Source: CAD feature listing. Evaluate the final solid. Frame: model axes, mm. Give positions to 0.01 mm unless a question says otherwise; leave off trailing zeros. Use CSV: the item, a comma, the result in double quotes.
```python
from build123d import *

# Parameters (mm, degrees)
EXTRUDE_1_DEPTH     = 15
SKETCH_2_R          = 0.75
CUT_EXTRUDE_1_DEPTH = 15
SKETCH_3_R          = 0.75
CUT_EXTRUDE_2_DEPTH = 15
CUT_EXTRUDE_START   = -2.7
SKETCH_2_2_R        = 0.75
CUT_EXTRUDE_3_DEPTH = 1
CUT_EXTRUDE_3_TAPER = -60
CUT_EXTRUDE_START_2 = 2.7
SKETCH_3_2_R        = 0.75
CUT_EXTRUDE_4_DEPTH = 1
CUT_EXTRUDE_4_TAPER = -60
FILLET_1_R          = 0.5


with BuildPart() as part:
    # Sketch 1 → Extrude 1 (new body)
    with BuildSketch(Plane(origin=(0, 0, 0), x_dir=(0, 0, -1), z_dir=(1, 0, 0))):
        with BuildLine():
            Line((0, 0), (-3, 0))
            Line((-3, 0), (-3, -20))
            Line((-3, -20), (-10.878462024, -21.389185421))
            Line((-10.878462024, -21.389185421), (-10.357517491, -24.34360868))
            Line((-10.357517491, -24.34360868), (-2.479055467, -22.954423259))
            ThreePointArc((-2.479055467, -22.954423259), (-0.701866671, -21.928362829), (0, -20))
            Line((0, -20), (0, 0))
        make_face()
    extrude(amount=EXTRUDE_1_DEPTH)

    # Sketch 2 → Cut-Extrude 1 (cut)
    with BuildSketch(Plane.XY.offset(3)):
        with Locations((2, -3)):
            Circle(SKETCH_2_R)
        with Locations((5.666666667, -3)):
            Circle(SKETCH_2_R)
        with Locations((9.333333333, -3)):
            Circle(SKETCH_2_R)
        with Locations((13, -3)):
            Circle(SKETCH_2_R)
        with Locations((3.680498092, -5.4)):
            Circle(SKETCH_2_R)
        with Locations((7.347164758, -5.4)):
            Circle(SKETCH_2_R)
        with Locations((11.013831425, -5.4)):
            Circle(SKETCH_2_R)
        with Locations((2, -7.8)):
            Circle(SKETCH_2_R)
        with Locations((5.666666667, -7.8)):
            Circle(SKETCH_2_R)
        with Locations((3.680498092, -10.2)):
            Circle(SKETCH_2_R)
        with Locations((7.347164758, -10.2)):
            Circle(SKETCH_2_R)
        with Locations((9.333333333, -7.8)):
            Circle(SKETCH_2_R)
        with Locations((11.013831425, -10.2)):
            Circle(SKETCH_2_R)
        with Locations((13, -7.8)):
            Circle(SKETCH_2_R)
        with Locations((2, -12.6)):
            Circle(SKETCH_2_R)
        with Locations((5.666666667, -12.6)):
            Circle(SKETCH_2_R)
        with Locations((3.680498092, -15)):
            Circle(SKETCH_2_R)
        with Locations((7.347164758, -15)):
            Circle(SKETCH_2_R)
        with Locations((9.333333333, -12.6)):
            Circle(SKETCH_2_R)
        with Locations((11.013831425, -15)):
            Circle(SKETCH_2_R)
        with Locations((13, -12.6)):
            Circle(SKETCH_2_R)
    extrude(amount=-CUT_EXTRUDE_1_DEPTH, mode=Mode.SUBTRACT)

    # Sketch 3 → Cut-Extrude 2 (cut)
    with BuildSketch(Plane(origin=(0, -23.26814693, 21.534582269), x_dir=(1, 0, 0), z_dir=(0, -0.984807753, -0.173648178))):
        with Locations((2, -13.820508076)):
            Circle(SKETCH_3_R)
        with Locations((5.666666667, -13.820508076)):
            Circle(SKETCH_3_R)
        with Locations((9.333333333, -13.820508076)):
            Circle(SKETCH_3_R)
        with Locations((13, -13.820508076)):
            Circle(SKETCH_3_R)
        with Locations((4.013839115, -16.220508076)):
            Circle(SKETCH_3_R)
        with Locations((7.680505781, -16.220508076)):
            Circle(SKETCH_3_R)
        with Locations((11.347172448, -16.220508076)):
            Circle(SKETCH_3_R)
    extrude(amount=CUT_EXTRUDE_2_DEPTH, mode=Mode.SUBTRACT)

    # Sketch 2_2 → Cut-Extrude 3 (cut)
    with BuildSketch(Plane.XY.offset(3).offset(CUT_EXTRUDE_START)):
        with Locations((2, -3)):
            Circle(SKETCH_2_2_R)
        with Locations((5.666666667, -3)):
            Circle(SKETCH_2_2_R)
        with Locations((9.333333333, -3)):
            Circle(SKETCH_2_2_R)
        with Locations((13, -3)):
            Circle(SKETCH_2_2_R)
        with Locations((3.680498092, -5.4)):
            Circle(SKETCH_2_2_R)
        with Locations((7.347164758, -5.4)):
            Circle(SKETCH_2_2_R)
        with Locations((11.013831425, -5.4)):
            Circle(SKETCH_2_2_R)
        with Locations((2, -7.8)):
            Circle(SKETCH_2_2_R)
        with Locations((5.666666667, -7.8)):
            Circle(SKETCH_2_2_R)
        with Locations((3.680498092, -10.2)):
            Circle(SKETCH_2_2_R)
        with Locations((7.347164758, -10.2)):
            Circle(SKETCH_2_2_R)
        with Locations((9.333333333, -7.8)):
            Circle(SKETCH_2_2_R)
        with Locations((11.013831425, -10.2)):
            Circle(SKETCH_2_2_R)
        with Locations((13, -7.8)):
            Circle(SKETCH_2_2_R)
        with Locations((2, -12.6)):
            Circle(SKETCH_2_2_R)
        with Locations((5.666666667, -12.6)):
            Circle(SKETCH_2_2_R)
        with Locations((3.680498092, -15)):
            Circle(SKETCH_2_2_R)
        with Locations((7.347164758, -15)):
            Circle(SKETCH_2_2_R)
        with Locations((9.333333333, -12.6)):
            Circle(SKETCH_2_2_R)
        with Locations((11.013831425, -15)):
            Circle(SKETCH_2_2_R)
        with Locations((13, -12.6)):
            Circle(SKETCH_2_2_R)
    extrude(amount=-CUT_EXTRUDE_3_DEPTH, taper=CUT_EXTRUDE_3_TAPER, mode=Mode.SUBTRACT)

    # Sketch 3_2 → Cut-Extrude 4 (cut)
    with BuildSketch(Plane(origin=(0, -23.26814693, 21.534582269), x_dir=(1, 0, 0), z_dir=(0, -0.984807753, -0.173648178)).offset(CUT_EXTRUDE_START_2)):
        with Locations((2, -13.820508076)):
            Circle(SKETCH_3_2_R)
        with Locations((5.666666667, -13.820508076)):
            Circle(SKETCH_3_2_R)
        with Locations((9.333333333, -13.820508076)):
            Circle(SKETCH_3_2_R)
        with Locations((13, -13.820508076)):
            Circle(SKETCH_3_2_R)
        with Locations((4.013839115, -16.220508076)):
            Circle(SKETCH_3_2_R)
        with Locations((7.680505781, -16.220508076)):
            Circle(SKETCH_3_2_R)
        with Locations((11.347172448, -16.220508076)):
            Circle(SKETCH_3_2_R)
    extrude(amount=CUT_EXTRUDE_4_DEPTH, taper=CUT_EXTRUDE_4_TAPER, mode=Mode.SUBTRACT)

    # Fillet 1
    fillet_1_edges = [part.edges().sort_by_distance(p)[0] for p in [
        (0, -10, 0),
        (7.5, -24.34360868, 10.357517491),
        (15, -10, 3),
        (7.5, -21.389185421, 10.878462024),
        (7.5, -20, 3),
        (7.5, 0, 3),
        (7.5, 0, 0),
        (15, -20.694592711, 6.939231012),
        (15, -22.866397051, 10.617989758),
        (15, -23.64901597, 6.418286479),
        (15, -21.928362829, 0.701866671),
        (15, -10, 0),
        (0, -21.928362829, 0.701866671),
        (0, -23.64901597, 6.418286479),
        (0, -22.866397051, 10.617989758),
        (0, -20.694592711, 6.939231012),
        (15, 0, 1.5),
        (0, -10, 3),
        (0, 0, 1.5),
    ]]
    fillet(fillet_1_edges, radius=FILLET_1_R)


solid = part.part
```
1. Pin query (flat end, axial travel): P1, Ø1.5, axis at x = 4.5, z = 2.5, coming from the -Y side; P2, Ø7, axis at x = 4, y = -6.5, coming from the +Z side; P3, Ø3, axis at x = 6, z = 8.5, coming from the +Y side. Return the tip coordinate at first contact, or that it passes through.
Answer below:
P1,"stops at y = -23.09"
P2,"stops at z = 3"
P3,"stops at y = -20.71"
2. Ray query, line 1 along X through (y, z) = (-3, 1.55); line 2 along X through (y, z) = (-15, 0.9); line 3 along Y through (x, z) = (13, 0.95). Return the intervals inside material, ascending.
Answer below:
line 1,"x = 0 to 1.25, 2.75 to 4.92, 6.42 to 8.58, 10.08 to 12.25, 13.75 to 15"
line 2,"x = 0 to 2.93, 4.43 to 6.6, 8.1 to 10.26, 11.76 to 15"
line 3,"y = -22.19 to -13.35, -11.85 to -8.55, -7.05 to -3.75, -2.25 to 0"
3. Mould query, pull axis Y, two halves, no side actions, for faces 1 (the cylindrical face through (0.15, -23.456, 6.145)), 2 (the flat face through (0, -14, 2)), 3 (the cylindrical face through (11.36, -6.065, 1.669)). Classes: released by +Y, released by -Y, zero draft, split by the parting line, or undercut.
Answer below:
face 1,"released by -Y"
face 2,"zero draft"
face 3,"undercut"
4. Section query A-A on y = -10.2. Count the separate pieces of the cut face and the enclosed holes in it, plus the area to 3 significant figures.
Answer below:
separate pieces,"4"
enclosed holes,"0"
area,"30.8 mm²"
